Source: CAD feature listing. Evaluate the final solid. Frame: model axes, mm. Face numbers are marked on the shaded views. A direction names the side the tool comes from. Coordinates: 2 decimals unless noted, no trailing zeros. Order: outer loops, then holes, each group sorted by start corner. A loop starts at its lowest first (then second) coordinate and runs counter-clockwise, first axis right, second up.
Item 1: Mould query, pull axis X, two halves, no side actions, for the marked faces 6, 7 and 8. Classes: released by +X, released by -X, zero draft, split by the parting line, or undercut.
Item 2: Section D-D on y = 1.5. Return the cut outline in (x, z).
Item 3: Reachability of the marked faces 1, 2, 3, 4 and 5 from +Z, -Z, +X, -X, +Y, -Y: full face, straight path, thin tool, end or side. Return the list, or none.
Item 4: Section A-A on y = 8. Return the cut outline in (x, z), then the cut area to 3 significant figures.
Item 5: Section B-B on x = -2.5. Return the cut outline in (y, z), then the cut area to 3 significant figures.
Item 6: Contact query for flat-ended pins moving along their axis: P1, Ø6.5, axis at x = 6, y = 7, coming from the -Z side; P2, Ø1.6, axis at y = 0.5, z = 5.5, coming from the +X side; P3, Ø1, axis at y = 5, z = 1, coming from the +X side. Output: stop coordinate, or through.
Item 7: Ray query, line 1 (Z direction, x = 12.5, y = 10); line 2 (Z direction, x = 0.5, y = 10); line 3 (X direction, y = 5.75, z = -0.5). Return the intervals inside material, ascending.
Item 8: Section C-C on z = -10.5. Return the cut outline in (x, y).
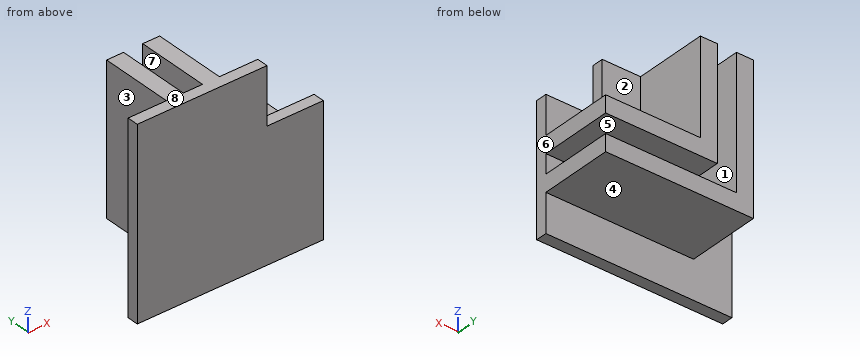
from build123d import *

# Parameters (mm, degrees)
ESQUISSE1_W              = 13
ESQUISSE1_H              = 20
BOSS_EXTRU_1_DEPTH       = 15
ESQUISSE2_W              = 2
ESQUISSE2_H              = 20
ESQUISSE2_W_2            = 3
ENL_V_MAT_EXTRU_2_DEPTH  = 13
ESQUISSE4_W              = 20
ESQUISSE4_H              = 2
BOSS_EXTRU_2_DEPTH       = 5
ESQUISSE5_W              = 20
ESQUISSE5_H              = 2
BOSS_EXTRU_3_DEPTH       = 5
ESQUISSE6_W              = 20
ESQUISSE6_H              = 13
ENL_V_MAT_EXTRU_3_DEPTH  = 0.2
ESQUISSE7_W              = 20
ESQUISSE7_H              = 13
ENL_V_MAT_EXTRU_4_DEPTH  = 0.2
ESQUISSE8_W              = 20
ESQUISSE8_H              = 13
BOSS_EXTRU_4_DEPTH       = 0.2
ESQUISSE9_W              = 20
ESQUISSE9_H              = 13
BOSS_EXTRU_5_DEPTH       = 0.2
ENL_V_MAT_EXTRU_5_DEPTH  = 10
BOSS_EXTRU_6_DEPTH       = 2
ESQUISSE13_W             = 3
ESQUISSE13_H             = 23
BOSS_EXTRU_7_DEPTH       = 13
ESQUISSE14_W             = 16.8
ESQUISSE14_H             = 3
ESQUISSE14_W_2           = 16.2
BOSS_EXTRU_8_DEPTH       = 13
ESQUISSE18_W             = 3.4
ESQUISSE18_H             = 13
ENL_V_MAT_EXTRU_8_DEPTH  = 10
ESQUISSE19_W             = 6.8
ESQUISSE19_H             = 13
ENL_V_MAT_EXTRU_9_DEPTH  = 10
ESQUISSE20_W             = 6.8
ESQUISSE20_H             = 13
ENL_V_MAT_EXTRU_10_DEPTH = 10
ESQUISSE21_W             = 3.4
ESQUISSE21_H             = 13
ENL_V_MAT_EXTRU_11_DEPTH = 5


with BuildPart() as part:
    # Esquisse1 → Boss.-Extru.1 (new body)
    with BuildSketch(Plane(origin=(0, 0, 0), x_dir=(1, 0, 0), z_dir=(0, 1, 0))):
        with Locations((-1.892857143, 1.160714286)):
            Rectangle(ESQUISSE1_W, ESQUISSE1_H)
    extrude(amount=BOSS_EXTRU_1_DEPTH)

    # Esquisse2 → Enlèv. mat.-Extru.2 (cut)
    with BuildSketch(Plane(origin=(0, 15, 0), x_dir=(1, 0, 0), z_dir=(0, 1, 0))):
        with Locations((-7.392857143, 1.160714286)):
            Rectangle(ESQUISSE2_W, ESQUISSE2_H)
        with Locations((-1.892857143, 1.160714286)):
            Rectangle(ESQUISSE2_W_2, ESQUISSE2_H)
        with Locations((3.607142857, 1.160714286)):
            Rectangle(ESQUISSE2_W, ESQUISSE2_H)
    extrude(amount=-ENL_V_MAT_EXTRU_2_DEPTH, mode=Mode.SUBTRACT)

    # Esquisse4 → Boss.-Extru.2 (add)
    with BuildSketch(Plane.ZY.offset(8.392857143)):
        with Locations((-1.160714286, 1)):
            Rectangle(ESQUISSE4_W, ESQUISSE4_H)
    extrude(amount=BOSS_EXTRU_2_DEPTH)

    # Esquisse5 → Boss.-Extru.3 (add)
    with BuildSketch(Plane(origin=(4.607142857, 0, 0), x_dir=(0, 0, -1), z_dir=(1, 0, 0))):
        with Locations((1.160714286, 1)):
            Rectangle(ESQUISSE5_W, ESQUISSE5_H)
    extrude(amount=BOSS_EXTRU_3_DEPTH)

    # Esquisse6 → Enlèv. mat.-Extru.3 (cut)
    with BuildSketch(Plane.ZY.offset(0.392857143)):
        with Locations((-1.160714286, 8.5)):
            Rectangle(ESQUISSE6_W, ESQUISSE6_H)
    extrude(amount=-ENL_V_MAT_EXTRU_3_DEPTH, mode=Mode.SUBTRACT)

    # Esquisse7 → Enlèv. mat.-Extru.4 (cut)
    with BuildSketch(Plane(origin=(-3.392857143, 0, 0), x_dir=(0, 0, -1), z_dir=(1, 0, 0))):
        with Locations((1.160714286, 8.5)):
            Rectangle(ESQUISSE7_W, ESQUISSE7_H)
    extrude(amount=-ENL_V_MAT_EXTRU_4_DEPTH, mode=Mode.SUBTRACT)

    # Esquisse8 → Boss.-Extru.4 (add)
    with BuildSketch(Plane(origin=(2.607142857, 0, 0), x_dir=(0, 0, -1), z_dir=(1, 0, 0))):
        with Locations((1.160714286, 8.5)):
            Rectangle(ESQUISSE8_W, ESQUISSE8_H)
    extrude(amount=BOSS_EXTRU_4_DEPTH)

    # Esquisse9 → Boss.-Extru.5 (add)
    with BuildSketch(Plane.ZY.offset(6.392857143)):
        with Locations((-1.160714286, 8.5)):
            Rectangle(ESQUISSE9_W, ESQUISSE9_H)
    extrude(amount=BOSS_EXTRU_5_DEPTH)

    # Esquisse11 → Enlèv. mat.-Extru.5 (cut)
    with BuildSketch(Plane(origin=(0, 0, -11.160714286), x_dir=(-1, 0, 0), z_dir=(0, 0, -1))):
        Polygon((6.592857143, 2), (6.592857143, 15), (3.592857143, 15), (3.592857143, 2), (0.192857143, 2), (0.192857143, 15), (-2.807142857, 15), (-2.807142857, 2), (-9.607142857, 2), (-9.607142857, 0), (13.392857143, 0), (13.392857143, 2), align=None)
    extrude(amount=-ENL_V_MAT_EXTRU_5_DEPTH, mode=Mode.SUBTRACT)

    # Esquisse12 → Boss.-Extru.6 (add)
    with BuildSketch(Plane(origin=(0, 0, 0), x_dir=(1, 0, 0), z_dir=(0, 1, 0))):
        Polygon((9.607142857, 1.160714286), (19.607142857, 1.160714286), (19.607142857, 24.160714286), (-13.392857143, 24.160714286), (-13.392857143, 1.160714286), align=None)
    extrude(amount=BOSS_EXTRU_6_DEPTH)

    # Esquisse13 → Boss.-Extru.7 (add)
    with BuildSketch(Plane(origin=(0, 2, 0), x_dir=(1, 0, 0), z_dir=(0, 1, 0))):
        Polygon((2.807142857, 1.160714286), (-0.192857143, 1.160714286), (-0.192857143, 24.160714286), (2.807142857, 24.160714286), (2.807142857, 1.789853377), align=None)
        with Locations((-5.092857143, 12.660714286)):
            Rectangle(ESQUISSE13_W, ESQUISSE13_H)
    extrude(amount=BOSS_EXTRU_7_DEPTH)

    # Esquisse14 → Boss.-Extru.8 (add)
    with BuildSketch(Plane(origin=(0, 2, 0), x_dir=(1, 0, 0), z_dir=(0, 1, 0))):
        with Locations((11.207142857, 9.460714286)):
            Rectangle(ESQUISSE14_W, ESQUISSE14_H)
        with Locations((11.207142857, 15.860714286)):
            Rectangle(ESQUISSE14_W, ESQUISSE14_H)
        with Locations((-5.292857143, 9.460714286)):
            Rectangle(ESQUISSE14_W_2, ESQUISSE14_H)
        with Locations((-5.292857143, 15.860714286)):
            Rectangle(ESQUISSE14_W_2, ESQUISSE14_H)
    extrude(amount=BOSS_EXTRU_8_DEPTH)

    # Esquisse18 → Enlèv. mat.-Extru.8 (cut)
    with BuildSketch(Plane(origin=(0, 0, -10.960714286), x_dir=(-1, 0, 0), z_dir=(0, 0, -1))):
        with Locations((1.892857143, 8.5)):
            Rectangle(ESQUISSE18_W, ESQUISSE18_H)
    extrude(amount=-ENL_V_MAT_EXTRU_8_DEPTH, mode=Mode.SUBTRACT)

    # Esquisse19 → Enlèv. mat.-Extru.9 (cut)
    with BuildSketch(Plane(origin=(0, 0, -17.360714286), x_dir=(-1, 0, 0), z_dir=(0, 0, -1))):
        with Locations((9.992857143, 8.5)):
            Rectangle(ESQUISSE19_W, ESQUISSE19_H)
    extrude(amount=-ENL_V_MAT_EXTRU_9_DEPTH, mode=Mode.SUBTRACT)

    # Esquisse20 → Enlèv. mat.-Extru.10 (cut)
    with BuildSketch(Plane(origin=(2.807142857, 0, 0), x_dir=(0, 0, -1), z_dir=(1, 0, 0))):
        with Locations((20.760714286, 8.5)):
            Rectangle(ESQUISSE20_W, ESQUISSE20_H)
    extrude(amount=-ENL_V_MAT_EXTRU_10_DEPTH, mode=Mode.SUBTRACT)

    # Esquisse21 → Enlèv. mat.-Extru.11 (cut)
    with BuildSketch(Plane(origin=(2.807142857, 0, 0), x_dir=(0, 0, -1), z_dir=(1, 0, 0))):
        with Locations((12.660714286, 8.5)):
            Rectangle(ESQUISSE21_W, ESQUISSE21_H)
    extrude(amount=-ENL_V_MAT_EXTRU_11_DEPTH, mode=Mode.SUBTRACT)


solid = part.part
Answer list:
1. face 6: released by +X
1. face 7: undercut
1. face 8: zero draft
2. outline: (-13.39, -24.16) - (19.61, -24.16) - (19.61, -1.16) - (9.61, -1.16) - (9.61, 8.84) - (-13.39, 8.84) - close
3. face 1: +Z, +Y
3. face 2: +Z, +X, +Y
3. face 3: +Z, -Z, -X, +Y
3. face 4: -Z, +X, -X, +Y
3. face 5: +X, +Y
4. outline: (-6.59, -17.36) - (19.61, -17.36) - (19.61, -14.36) - (-3.59, -14.36) - (-3.59, 8.84) - (-6.59, 8.84) - close; (-0.19, -10.96) - (19.61, -10.96) - (19.61, -7.96) - (2.81, -7.96) - (2.81, 8.84) - (-0.19, 8.84) - close
4. area: 258 mm2
5. outline: (0, -24.16) - (2, -24.16) - (2, -17.36) - (15, -17.36) - (15, -14.36) - (2, -14.36) - (2, 8.84) - (0, 8.84) - close
5. area: 105 mm2
6. P1: stops at z = -17.36
6. P2: stops at x = 9.61
6. P3: stops at x = 2.81
7. line 1: z = -17.36 to -14.36, -10.96 to -7.96
7. line 2: z = -17.36 to -14.36, -10.96 to 8.84
7. line 3: x = -6.59 to -3.59, -0.19 to 2.81
8. outline: (-13.39, 0) - (19.61, 0) - (19.61, 15) - (-0.19, 15) - (-0.19, 2) - (-3.59, 2) - (-3.59, 15) - (-6.59, 15) - (-6.59, 2) - (-13.39, 2) - close
